The model under review builds one solid part; all positions refer to its coordinate system, in mm. A direction names the side the tool comes from. Give positions to 0.01 mm unless a question says otherwise; leave off trailing zeros. Loops run counter-clockwise (first coordinate to the right, second up) from the corner with the lowest first, then second, coordinate; pieces in that order, holes last. Notation, with made-up numbers: (-22.75, 8) -> (29.25, 8) arc R11 ccw to (29.25, 28) -> close; hole circle Ø8 at (70.25, 76.25). An arc over 180 degrees is marked (long way). Write each question's results on one line, items separated by ' | '. Start each with the question number.
Q1. Mouldability with a two-part tool opening along X and no side actions: class faces 1 (the face through (8.05, 1.09, 8.84)), 2 (the face through (0, 17, 1)), 3 (the face through (8, 40.64, 1)) as released by +X, released by -X, zero draft, split by the parting line, or undercut.
Q2. We need section B-B (x = 5.75). Write out the cut boundary in (y, z).
Q3. We need section C-C (z = 8). Write out the cut boundary in (x, y).
Q4. Wall thickness on L1, parallel to Y at x = 8.5, z = 12.25: over which ranges is the line inside the solid? List them lowest first. Write a range as [from, to].
Q5. Insertion check: pin 1 Ø5 at (x, y) = (3.5, 34) entering from +Z; pin 2 Ø4 at (x, z) = (5.5, 9) entering from +Y. Each pin has a flat end and moves straight along its axis. Give the tip position at first contact, or say it passes through.
Q6. Machinability: for faces 4 (the face through (8, 22, 2.159)), 5 (the face through (8, 1, 13.589)), which of the approach directions +Z, -Z, +X, -X, +Y, -Y give a long, thin tool a straight path to every point of the face, cutting with its end or side? Answer none if there is none.
Q7. We need section A-A (x = 7.5). Write out the cut boundary in (y, z).
Autodesk Inventor part; units mm, degrees
ref_plane "YZ Plane" through (0, 0, 0) normal (1, 0, 0) x (0, 1, 0)
ref_plane "XZ Plane" through (0, 0, 0) normal (0, 1, 0) x (-1, 0, 0)
ref_plane "XY Plane" through (0, 0, 0) normal (0, 0, 1) x (1, 0, 0)
sketch "Sketch1" plane through (0, 0, 0) normal (0, 0, 1) x (1, 0, 0)
  line L0 (0, 0) -> (16.51, 0)
  line L1 (16.51, 0) -> (16.51, 40.64)
  line L2 (16.51, 40.64) -> (0, 40.64)
  line L3 (0, 40.64) -> (0, 0)
  dimension "d0" = 40.64
  dimension "d1" = 16.51
extrude "Extrusion1" add sketch "Sketch1" along normal blind 2.159
sketch "Sketch2" plane through (0, 0, 2.159) normal (0, 0, 1) x (1, 0, 0)
  line L0 (0, 0) -> (16.51, 0)
  line L1 (16.51, 0) -> (16.51, 40.64)
  line L2 (0, 0) -> (16.51, 0)
  line L3 (16.51, 0) -> (16.51, 2.159)
  line L4 (16.51, 2.159) -> (0, 2.159)
  line L5 (0, 2.159) -> (0, 0)
  dimension "d4" = 2.159
extrude "Extrusion2" add sketch "Sketch2" along normal blind 11.43
sketch "Sketch3" plane through (0, 2.159, 2.159) normal (0, 1, 0) x (1, 0, 0)
  circle A0 centre (8.255, -8.255) radius 1.5875
  line L0 (16.51, -11.43) -> (0, -11.43)
  point P0 (0, 2.159)
  dimension "d8" = 3.175
  dimension "d12" = 3.175
extrude "Extrusion3" cut sketch "Sketch3" against normal blind 11.43
properties part number "L Bracket" material "Steel, Galvanized"
Output:
1) face 1: undercut | face 2: released by -X | face 3: zero draft
2) outline: (0, 0) -> (40.64, 0) -> (40.64, 2.16) -> (2.16, 2.16) -> (2.16, 13.59) -> (0, 13.59) -> close
3) outline: (0, 0) -> (16.51, 0) -> (16.51, 2.16) -> (0, 2.16) -> close
4) L1: [0, 2.16]
5) pin 1: z = 2.16 | pin 2: y = 2.16
6) face 4: +Z, +X, -X, +Y | face 5: +Z, +X, -X, +Y, -Y
7) outline: (0, 0) -> (40.64, 0) -> (40.64, 2.16) -> (2.16, 2.16) -> (2.16, 9.02) -> (0, 9.02) -> close; (0, 11.81) -> (2.16, 11.81) -> (2.16, 13.59) -> (0, 13.59) -> close
